Build history of the part. All positions in model axes, mm. Face numbers are marked on the shaded views. A direction names the side the tool comes from. Coordinates: 2 decimals unless noted, no trailing zeros. Loops run counter-clockwise (first coordinate to the right, second up) from the corner with the lowest first, then second, coordinate; pieces in that order, holes last. Notation, with made-up numbers: (33, 87.5) - (91, 87.5) arc R28 ccw to (91, 117.5) - close; hole circle Ø9 at (-11.5, -33.5). An arc over 180 degrees is marked (long way). One line per item, written item: value.
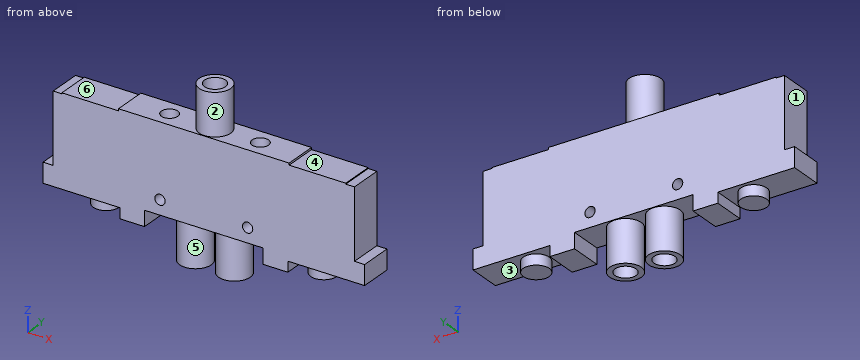
```python
from build123d import *

# Parameters (mm, degrees)
SKETCH1_R                       = 1.5875
BOSS_EXTRUDE1_DEPTH             = 10.2235
SKETCH2_R                       = 4.88315
SKETCH2_R_2                     = 3.2512
BOSS_EXTRUDE2_DEPTH             = 12.954
SKETCH3_R                       = 4.88315
SKETCH3_R_2                     = 3.2512
BOSS_EXTRUDE3_DEPTH             = 12.954
TAP_DRILL_FOR_1_4_20_TAP1_D     = 5.1054
TAP_DRILL_FOR_1_4_20_TAP1_DEPTH = 9.0551
TAP_DRILL_FOR_1_4_20_TAP1_TIP   = 1.533816902
SKETCH6_R                       = 4.0005
BOSS_EXTRUDE4_DEPTH             = 3.2512


with BuildPart() as part:
    # Sketch1 → Boss-Extrude1 (new body)
    with BuildSketch(Plane(origin=(0, 0, 0), x_dir=(1, 0, 0), z_dir=(0, 1, 0))):
        Polygon((-18.3007, 0), (18.3007, 0), (18.3007, 4.7498), (25.9207, 4.7498), (25.9207, 1.5367), (49.6316, 1.5367), (49.6316, -4.5593), (46.4947, -4.5593), (46.4947, -26.1239), (43.815, -26.1239), (43.815, -26.4033), (26.3398, -26.4033), (26.3398, -27.0129), (-26.3398, -27.0129), (-26.3398, -26.4033), (-43.815, -26.4033), (-43.815, -26.1239), (-46.4947, -26.1239), (-46.4947, -4.5593), (-49.6316, -4.5593), (-49.6316, 1.5367), (-25.9207, 1.5367), (-25.9207, 4.7498), (-18.3007, 4.7498), align=None)
        with Locations(Location((13.5255, -4.4577, 0), (0, 0, 270))):
            Circle(SKETCH1_R, mode=Mode.SUBTRACT)
        with Locations(Location((-13.5255, -4.4577, 0), (0, 0, 90))):
            Circle(SKETCH1_R, mode=Mode.SUBTRACT)
    extrude(amount=BOSS_EXTRUDE1_DEPTH)

    # Sketch2 → Boss-Extrude2 (add)
    with BuildSketch(Plane.XY.offset(27.0129)):
        with Locations(Location((0, 5.11175, 0), (0, 0, 180))):
            Circle(SKETCH2_R)
        with Locations((0, 5.11175)):
            Circle(SKETCH2_R_2, mode=Mode.SUBTRACT)
    extrude(amount=BOSS_EXTRUDE2_DEPTH)

    # Sketch3 → Boss-Extrude3 (add)
    # profile 1 of 2: a face of its own
    with BuildSketch(Plane(origin=(0, 0, 0), x_dir=(-1, 0, 0), z_dir=(0, 0, -1))):
        with Locations(Location((6.0071, 5.11175, 0), (0, 0, 180))):
            Circle(SKETCH3_R)
        with Locations((6.0071, 5.11175)):
            Circle(SKETCH3_R_2, mode=Mode.SUBTRACT)
    # profile 2 of 2: a face of its own
    with BuildSketch(Plane(origin=(0, 0, 0), x_dir=(-1, 0, 0), z_dir=(0, 0, -1))):
        with Locations(Location((-6.0071, 5.11175, 0), (0, 0, 180))):
            Circle(SKETCH3_R)
        with Locations((-6.0071, 5.11175)):
            Circle(SKETCH3_R_2, mode=Mode.SUBTRACT)
    extrude(amount=BOSS_EXTRUDE3_DEPTH)

    # Tap Drill for 1/4-20 Tap1
    with Locations(Plane.XY.offset(27.0129)):
        with Locations((-13.9954, 5.11175), (13.9954, 5.11175)):
            Hole(TAP_DRILL_FOR_1_4_20_TAP1_D / 2, depth=TAP_DRILL_FOR_1_4_20_TAP1_DEPTH)
            with Locations((0, 0, -(TAP_DRILL_FOR_1_4_20_TAP1_DEPTH + TAP_DRILL_FOR_1_4_20_TAP1_TIP / 2))):  # 118° drill point
                Cone(0, TAP_DRILL_FOR_1_4_20_TAP1_D / 2, TAP_DRILL_FOR_1_4_20_TAP1_TIP, mode=Mode.SUBTRACT)

    # Sketch6 → Boss-Extrude4 (add)
    with BuildSketch(Plane(origin=(0, 0, -1.5367), x_dir=(-1, 0, 0), z_dir=(0, 0, -1))):
        with Locations(Location((-33.5661, 5.11175, 0), (0, 0, 180))):
            Circle(SKETCH6_R)
        with Locations(Location((33.5661, 5.11175, 0), (0, 0, 180))):
            Circle(SKETCH6_R)
    extrude(amount=BOSS_EXTRUDE4_DEPTH)


solid = part.part
```
Item 1: Cut at B-B, the plane z = 10. Write the cut outline in (x, y), then the cut area to 3 significant figures.
Check result:
outline: (-46.49, 0) - (46.49, 0) - (46.49, 10.22) - (-46.49, 10.22) - close
area: 951 mm^2
Item 2: Drop flat-ended pins along their axis: P1, Ø1.4, axis at y = 5, z = -3, coming from the +X side; P2, Ø5, axis at x = -39, y = 4, coming from the -Z side; P3, Ø4, axis at y = 3, z = 25.5, coming from the +X side; P4, Ø2.5, axis at x = -13.53, z = 4.46, coming from the -Y side. Give the stop position or say it passes through.
Check result:
P1: stops at x = 37.57
P2: stops at z = -4.79
P3: stops at x = 46.49
P4: passes through
Item 3: Tool access for the marked faces 4, 5 and 6: list every direction of +Z, -Z, +X, -X, +Y, -Y with a clear straight run to the whole face (end or side of a thin tool).
Check result:
face 4: +Z, +X, +Y, -Y
face 5: -Z
face 6: +Z, -X, +Y, -Y
Item 4: Cut at A-A, the plane x = 0. Write the cut outline in (y, z), then the cut area to 3 significant figures.
Check result:
outline: (0, 0) - (10.22, 0) - (10.22, 27.01) - (9.99, 27.01) - (9.99, 39.97) - (8.36, 39.97) - (8.36, 27.01) - (1.86, 27.01) - (1.86, 39.97) - (0.23, 39.97) - (0.23, 27.01) - (0, 27.01) - close
area: 318 mm^2
Item 5: Cut at D-D, the plane y = 6.5. Give the number of separate pieces and of enclosed holes in the cut face, then the cut area to 3 significant figures.
Check result:
separate pieces: 1
enclosed holes: 2
area: 2,750 mm^2
Item 6: Probe probe 1 along X at (y, z) = (1.5, -0.5); probe 2 along Z at (x, y) = (-18.5, 1.5); probe 3 along Y at (x, z) = (0, 33.75). List the from-to ranges inside material, lowest first. Write a range as from..to.
Check result:
probe 1: x = -49.63..-18.3, -9.29..-2.72, 2.72..9.29, 18.3..49.63
probe 2: z = -4.75..27.01
probe 3: y = 0.23..1.86, 8.36..9.99
Item 7: Cut at C-C, the plane z = 19.5. Write the cut outline in (x, y).
Check result:
outline: (-46.49, 0) - (46.49, 0) - (46.49, 10.22) - (-46.49, 10.22) - close; hole circle Ø5.11 at (-14, 5.11); hole circle Ø5.11 at (14, 5.11)
Item 8: Pull direction X, two halves, no side cores. Call the marked faces 1, 2 and 3: released by +X, released by -X, zero draft, split by the parting line, or undercut.
Check result:
face 1: released by -X
face 2: split by the parting line
face 3: undercut
